The model under review builds one solid part; all positions refer to its coordinate system, in mm. A direction names the side the tool comes from. Round coordinates to 2 decimals unless told otherwise and drop trailing zeros. Write each loop counter-clockwise with the first axis right and the second up, starting at its lowest first coordinate (ties: lowest second). Pieces come first, ordered by that corner, then holes. Notation, with made-up numbers: (80, 31) -> (118, 31) arc R27 ccw to (118, 49) -> close; hole circle Ø9 at (42, 20). An arc over 180 degrees is marked (long way). Answer as a JSON object with one key per item and string values. Group by question number.
1) We need section A-A, the plane x = 9.5. Write out the cut boundary in (y, z), then the cut area to 3 significant figures.
2) To check wall thickness, follow probe 1 along Z at (x, y) = (-18.5, 80); probe 2 along Y at (x, z) = (76, -7); probe 3 along Y at (x, z) = (0, 3.5). State the ranges of each line that lie inside material, in increasing order. Write a range as [from, to].
3) We need section B-B, the plane z = -10. Write out the cut boundary in (x, y), then the cut area to 3 significant figures.
4) Insertion check: pin 1 Ø10.5 at (x, z) = (80, 0) entering from +Y; pin 2 Ø13 at (y, z) = (80, 0) entering from -X; pin 3 Ø4 at (x, z) = (-67, 6) entering from -Y. Each pin has a flat end and moves straight along its axis. Give the tip position at first contact, or say it passes through.
5) We need section C-C, the plane y = 11. Write out the cut boundary in (x, z).
6) We need section D-D, the plane x = 80. Write out the cut boundary in (y, z), then the cut area to 3 significant figures.
7) Machinability: for faces 1 (the flat face through (0, -60, 0)), 2 (the flat face through (-85, -5, 0)), 3 (the flat face through (75, -5, 0)), which of the approach directions +Z, -Z, +X, -X, +Y, -Y give a long, thin tool a straight path to every point of the face, cutting with its end or side? Answer none if there is none.
from build123d import *

# Parameters (mm, degrees)
SKETCH1_R               = 100
SKETCH1_R_2             = 25
BOSS_EXTRUDE1_DEPTH     = 15
CUT_EXTRUDE1_DEPTH      = 12.5
CUT_EXTRUDE2_DEPTH      = 25
CUT_EXTRUDE2_DEPTH_BACK = 100
SKETCH3_R               = 4
CUT_EXTRUDE3_DEPTH      = 100
CUT_EXTRUDE3_DEPTH_BACK = 25
SKETCH4_R               = 4
CUT_EXTRUDE4_DEPTH      = 25
CUT_EXTRUDE4_DEPTH_BACK = 100
SKETCH5_R               = 4
CUT_EXTRUDE5_DEPTH      = 100
CUT_EXTRUDE5_DEPTH_BACK = 25
SKETCH6_R               = 4


with BuildPart() as part:
    # Sketch1 → Boss-Extrude1 (new, symmetric)
    with BuildSketch(Plane.XY):
        Circle(SKETCH1_R)
        Circle(SKETCH1_R_2, mode=Mode.SUBTRACT)
    extrude(amount=BOSS_EXTRUDE1_DEPTH, both=True)

    # Sketch2 → Cut-Extrude1 (cut, symmetric)
    with BuildSketch(Plane.XY):
        Polygon((60, -5), (110, -5), (100, 5), (60, 5), align=None)
        Polygon((-5, -60), (-5, -110), (5, -100), (5, -60), align=None)
        Polygon((-60, 5), (-110, 5), (-100, -5), (-60, -5), align=None)
        Polygon((5, 60), (5, 110), (-5, 100), (-5, 60), align=None)
    extrude(amount=CUT_EXTRUDE1_DEPTH, both=True, mode=Mode.SUBTRACT)

    # Sketch3 → Cut-Extrude2 (cut, two sides: drawn at the far end of the back side and taken through both)
    with BuildSketch(Plane(origin=(0, 0, 0), x_dir=(1, 0, 0), z_dir=(0, 1, 0)).offset(-CUT_EXTRUDE2_DEPTH_BACK)):
        with Locations(Location((80, 0, 0), (0, 0, 90))):
            Circle(SKETCH3_R)
    extrude(amount=CUT_EXTRUDE2_DEPTH + CUT_EXTRUDE2_DEPTH_BACK, mode=Mode.SUBTRACT)

    # Sketch4 → Cut-Extrude3 (cut, two sides: drawn at the far end of the back side and taken through both)
    with BuildSketch(Plane(origin=(0, 0, 0), x_dir=(0, 0, -1), z_dir=(1, 0, 0)).offset(-CUT_EXTRUDE3_DEPTH_BACK)):
        with Locations(Location((0, 80, 0), (0, 0, 180))):
            Circle(SKETCH4_R)
    extrude(amount=CUT_EXTRUDE3_DEPTH + CUT_EXTRUDE3_DEPTH_BACK, mode=Mode.SUBTRACT)

    # Sketch5 → Cut-Extrude4 (cut, two sides: drawn at the far end of the back side and taken through both)
    with BuildSketch(Plane(origin=(0, 0, 0), x_dir=(0, 0, -1), z_dir=(1, 0, 0)).offset(-CUT_EXTRUDE4_DEPTH_BACK)):
        with Locations(Location((0, -80, 0), (0, 0, 180))):
            Circle(SKETCH5_R)
    extrude(amount=CUT_EXTRUDE4_DEPTH + CUT_EXTRUDE4_DEPTH_BACK, mode=Mode.SUBTRACT)

    # Sketch6 → Cut-Extrude5 (cut, two sides: drawn at the far end of the back side and taken through both)
    with BuildSketch(Plane(origin=(0, 0, 0), x_dir=(1, 0, 0), z_dir=(0, 1, 0)).offset(-CUT_EXTRUDE5_DEPTH_BACK)):
        with Locations(Location((-80, 0, 0), (0, 0, 90))):
            Circle(SKETCH6_R)
    extrude(amount=CUT_EXTRUDE5_DEPTH + CUT_EXTRUDE5_DEPTH_BACK, mode=Mode.SUBTRACT)


solid = part.part
Here are the results:
{
 "1": {"outline": "(-99.55, -15) -> (-23.12, -15) -> (-23.12, 15) -> (-99.55, 15) -> close; (23.12, -15) -> (99.55, -15) -> (99.55, 15) -> (23.12, 15) -> close; hole circle Ø8 at (-80, 0); hole circle Ø8 at (80, 0)", "area": "4,480 mm^2"},
 "2": {"probe 1": "z = [-15, -4], [4, 15]", "probe 2": "y = [-64.99, -5], [5, 64.99]", "probe 3": "y = [-60, -25], [25, 60]"},
 "3": {"outline": "(-99.87, -5) arc R100 ccw to (-5, -99.87) -> (-5, -60) -> (5, -60) -> (5, -99.87) arc R100 ccw to (99.87, -5) -> (60, -5) -> (60, 5) -> (99.87, 5) arc R100 ccw to (5, 99.87) -> (5, 60) -> (-5, 60) -> (-5, 99.87) arc R100 ccw to (-99.87, 5) -> (-60, 5) -> (-60, -5) -> close; hole circle Ø50 at (0, 0)", "area": "27,900 mm^2"},
 "4": {"pin 1": "stops at y = 66.43", "pin 2": "stops at x = -67.81", "pin 3": "stops at y = -75.99"},
 "5": {"outline": "(-99.39, -15) -> (-22.45, -15) -> (-22.45, 15) -> (-99.39, 15) -> close; (22.45, -15) -> (99.39, -15) -> (99.39, 15) -> (22.45, 15) -> close; hole circle Ø8 at (-80, 0); hole circle Ø8 at (80, 0)"},
 "6": {"outline": "(-60, -15) -> (60, -15) -> (60, 15) -> (-60, 15) -> (-60, 4) -> (-5, 4) -> (-5, 12.5) -> (5, 12.5) -> (5, 4) -> (25, 4) -> (25, -4) -> (5, -4) -> (5, -12.5) -> (-5, -12.5) -> (-5, -4) -> (-60, -4) -> close", "area": "2,750 mm^2"},
 "7": {"face 1": "-Y", "face 2": "-X", "face 3": "+X"}
}
